Build history of the part. All positions in model axes, mm. A direction names the side the tool comes from. Coordinates: 2 decimals unless noted, no trailing zeros. Loops run counter-clockwise (first coordinate to the right, second up) from the corner with the lowest first, then second, coordinate; pieces in that order, holes last.
Item 1: Mould opens along X. For faces 4 (the face through (114.99, 21, -26)), 5 (the face through (47, 21, -72)), 6 (the face through (92.5, 6, -33)) say: released by +X, released by -X, zero draft, split by the parting line, or undercut.
Item 2: Drill centre lines: line 1 along X through (y, z) = (16.75, -8); line 2 along Z through (x, y) = (46.5, 35); line 3 along Z through (x, y) = (19.5, 8.5). Where is each one in solid material? Low to high.
Item 3: Cut at D-D (y = 25.5). List the corners of the cut face in (x, z).
Item 4: Cut at B-B (z = -14). List the corners of the cut face in (x, y), and give its area (3 significant figures).
Item 5: Cut at A-A (y = 8). List the corners of the cut face in (x, z), and give its area (3 significant figures).
Item 6: Cut at C-C (x = 23.5). List the corners of the cut face in (y, z), and give its area (3 significant figures).
Item 7: Flat gauge pins, fed straight in: pin 1 (1 mm diameter, centred on x = 28, z = -8, fed in from +Y); pin 2 (4 mm diameter, centred on x = 46.5, z = 3.5, fed in from -Y); pin 3 (2.5 mm diameter, centred on x = 0, z = -6, fed in from -Y). Where does each tip first touch, or does it go through?
Item 8: 3-axis set-ups, long thin cutter, end or side, ignore diameter. For faces 1 (the face through (-9.581, 3.042, -0.864)), 2 (the face through (88.026, 16.768, -57.481)), 3 (the face through (111.441, 33.234, -35.2)): which of +Z, -Z, +X, -X, +Y, -Y reach the whole face in a straight line?
Autodesk Inventor part; units mm, degrees
ref_plane "Work Plane2" through (0, 18, 0) normal (0, 1, 0) x (1, 0, 0)
ref_plane "YZ Plane" through (0, 0, 0) normal (1, 0, 0) x (0, 1, 0)
ref_plane "XZ Plane" through (0, 0, 0) normal (0, 1, 0) x (-1, 0, 0)
sketch "Sketch1" plane through (0, 0, 0) normal (0, 1, 0) x (-1, 0, 0)
  line L0 (0, 0) -> (-95, 0)
  line L1 (-95, 0) -> (-95, -65)
  line L2 (-95, -65) -> (0, -65)
  line L3 (0, -65) -> (0, 0)
  line L4 (0, -65) -> (12.9904, -57.5)
  line L5 (12.9904, -57.5) -> (12.9904, -7.5)
  line L6 (12.9904, -7.5) -> (0, 0)
  line L7 (-95, -65) -> (-107.9904, -57.5)
  line L8 (-107.9904, -57.5) -> (-107.9904, -7.5)
  line L9 (-107.9904, -7.5) -> (-95, 0)
  dimension "d0" = 95
  dimension "d1" = 65
  dimension "d2" = 15
  dimension "d3" = 15
  dimension "d4" = 120
  dimension "d5" = 15
  dimension "d6" = 15
  dimension "d7" = 120
extrude "Extrusion1" add sketch "Sketch1" along normal blind 5
sketch "Sketch2" plane through (0, 5, 0) normal (0, 1, 0) x (1, 0, 0)
  line L0 (1.0001, 63.5) -> (94.0001, 63.5)
  line L1 (94.0001, 63.5) -> (94.0001, 1.5)
  line L2 (94.0001, 1.5) -> (1.0001, 1.5)
  line L3 (1.0001, 1.5) -> (1.0001, 63.5)
  line L4 (0, 0) -> (95, 0)
  line L5 (-12.9904, 57.5) -> (-12.9904, 7.5)
  dimension "d10" = 93
  dimension "d11" = 62
  dimension "d12" = 1.5
  dimension "d13" = 13.9905
extrude "Extrusion2" add sketch "Sketch2" along normal blind 8
sketch "Sketch4" plane through (0, 5, 0) normal (0, 1, 0) x (1, 0, 0)
  line L0 (-12.9904, 57.5) -> (-12.9904, 7.5)
  line L1 (-12.9904, 57.5) -> (-12.9904, 7.5)
  line L2 (-12.9904, 7.5) -> (0, 0)
  line L3 (0, 0) -> (95, 0)
  line L4 (95, 0) -> (107.9904, 7.5)
  line L5 (95, 0) -> (107.9904, 7.5)
  line L6 (107.9904, 7.5) -> (107.9904, 57.5)
  line L7 (107.9904, 57.5) -> (95, 65)
  line L8 (107.9904, 57.5) -> (95, 65)
  line L9 (95, 65) -> (0, 65)
  line L10 (95, 65) -> (0, 65)
  line L11 (0, 65) -> (-12.9904, 57.5)
  line L12 (-19.9904, 61.5415) -> (-19.9904, 3.4585)
  line L13 (114.9904, 61.5415) -> (114.9904, 3.4585)
  line L14 (-1.8756, 72) -> (96.8756, 72)
  line L15 (-19.9904, 61.5415) -> (-1.8756, 72)
  line L16 (96.8756, 72) -> (114.9904, 61.5415)
  line L17 (114.9904, 3.4585) -> (96.8756, -7)
  line L18 (-19.9904, 3.4585) -> (-1.8756, -7)
  line L19 (-1.8756, -7) -> (96.8756, -7)
  line L20 (95, 0) -> (107.9904, 7.5)
  line L21 (107.9904, 7.5) -> (107.9904, 57.5)
  line L22 (0, 0) -> (95, 0)
  dimension "d22" = 7
  dimension "d23" = 7
  dimension "d24" = 7
  dimension "d25" = 7
  dimension "d26" = 7
  dimension "d27" = 7
  dimension "d28" = 7
  dimension "d29" = 7
extrude "Extrusion4" add sketch "Sketch4" along normal blind 32 and the other way blind 5
sketch "Sketch5" plane through (0, 0, 0) normal (0, -1, 0) x (1, 0, 0)
  line L0 (2.4999, -63) -> (92.4999, -63)
  line L1 (92.4999, -63) -> (92.4999, -2)
  line L2 (92.4999, -2) -> (2.4999, -2)
  line L3 (2.4999, -2) -> (2.4999, -63)
  line L4 (0, 0) -> (95, 0)
  line L5 (-12.9904, -57.5) -> (-12.9904, -7.5)
  line L6 (96.8756, 7) -> (-1.8756, 7)
  line L7 (114.9904, -61.5415) -> (114.9904, -3.4585)
  line L8 (-1.8756, -72) -> (96.8756, -72)
  dimension "d34" = 61
  dimension "d35" = 90
  dimension "d44" = 22.4905
  dimension "d128" = 9
extrude "Extrusion5" cut sketch "Sketch5" against normal blind 11
chamfer "Chamfer1" distance 6 angle 45 8 edges at (47.5, 0, -72) (105.933, 0, -66.7707) (114.9904, 0, -32.5) (105.933, 0, 1.7707) (47.5, 0, 7) (-10.933, 0, 1.7707) (-19.9904, 0, -32.5) (-10.933, 0, -66.7707)
sketch "Sketch6" plane through (0, 0, 0) normal (0, -1, 0) x (1, 0, 0)
  line L0 (2.4999, -2) -> (-2.5001, -2)
  line L1 (-2.5001, -2) -> (-2.5001, -63.0139)
  line L2 (-2.5001, -63.0139) -> (2.4999, -63.0139)
  line L3 (2.4999, -63.0139) -> (2.4999, -2)
  line L4 (2.4999, -2) -> (92.4999, -2)
  line L5 (92.4999, -2) -> (97.4999, -2)
  line L6 (97.4999, -2) -> (97.4999, -63.0139)
  line L7 (97.4999, -63.0139) -> (92.4999, -63.0139)
  line L8 (92.4999, -63.0139) -> (92.4999, -2)
  point P0 (0, 0)
  dimension "d45" = 5
  dimension "d46" = 5
extrude "Extrusion6" cut sketch "Sketch6" against normal blind 2
sketch "Sketch7" plane through (0, 2, 0) normal (0, -1, 0) x (1, 0, 0)
  circle A0 centre (-0.0001, -6) radius 1.6
  circle A1 centre (94.9999, -6) radius 1.6
  circle A2 centre (-0.0001, -59.0139) radius 1.6
  circle A3 centre (94.9999, -59.0139) radius 1.6
  line L0 (94.0001, -63.5) -> (94.0001, -1.5)
  line L1 (2.4999, -2) -> (2.4999, -63)
  line L2 (97.4999, -2) -> (97.4999, -63.0139)
  line L3 (-2.5001, -2) -> (97.4999, -2)
  line L4 (-2.5001, -63.0139) -> (-2.5001, -2)
  line L5 (2.4999, -63.0139) -> (-2.5001, -63.0139)
  line L6 (92.4999, -63) -> (92.4999, -2)
  line L7 (97.4999, -63.0139) -> (92.4999, -63.0139)
  point P0 (0, 0)
  dimension "d49" = 3.2
  dimension "d50" = 2.5
  dimension "d51" = 2.5
  dimension "d52" = 4
  dimension "d53" = 0
  dimension "d54" = 2.5
  dimension "d55" = 4
  dimension "d56" = 2.5
  dimension "d57" = 4
extrude "Extrusion7" cut sketch "Sketch7" against normal blind 1 contours A0 | A1 L0 | L0 A1 | L0 A3 | A3 L0 | A2
sketch "Sketch8" plane through (0, 13, 0) normal (0, 1, 0) x (1, 0, 0)
  line L0 (5.0001, 60.5) -> (90.0001, 60.5)
  line L1 (90.0001, 60.5) -> (90.0001, 4.5)
  line L2 (90.0001, 4.5) -> (5.0001, 4.5)
  line L3 (5.0001, 4.5) -> (5.0001, 60.5)
  line L4 (96.8756, 72) -> (-1.8756, 72)
  line L5 (-19.9904, 61.5415) -> (-19.9904, 3.4585)
  circle A0 centre (28.5001, 57) radius 2.5
  circle A1 centre (28.5001, 8) radius 2.5
  circle A2 centre (86.5001, 57) radius 2.5
  circle A3 centre (86.5001, 8) radius 2.5
  circle A4 centre (28.5001, 8) radius 1.6
  circle A5 centre (86.5001, 8) radius 1.6
  circle A6 centre (86.5001, 57) radius 1.6
  circle A7 centre (28.5001, 57) radius 1.6
  circle A8 centre (28.5001, 57) radius 2.5
  point P0 (0, 0)
  dimension "d60" = 85
  dimension "d61" = 56
  dimension "d62" = 11.5
  dimension "d63" = 24.9905
  dimension "d65" = 3.5
  dimension "d66" = 5
  dimension "d68" = 3.5
  dimension "d69" = 3.5
  dimension "d70" = 3.5
  dimension "d71" = 58
  dimension "d72" = 58
  dimension "d75" = 3.5
  dimension "d76" = 3.5
  dimension "d100" = 3.2
  dimension "d101" = 3.2
  dimension "d102" = 3.2
  dimension "d103" = 3.2
extrude "Extrusion8" add sketch "Sketch8" along normal blind 5 contours A0 | A1 | A2 | A3 | A4 | A5 | A6 | A7
sketch "Sketch9" plane through (92.4999, 11, -63) normal (-1, 0, 0) x (0, 0, 1)
  circle A0 centre (49, -3) radius 1.5
  line L0 (61, 0) -> (0, 0)
  line L1 (61, -9) -> (61, 0)
  point P0 (63, -11)
  dimension "d77" = 3
  dimension "d78" = 3
  dimension "d79" = 12
extrude "Extrusion9" cut sketch "Sketch9" against normal blind 5
sketch "Sketch10" plane through (0, 37, 0) normal (0, 1, 0) x (1, 0, 0)
  line L0 (-12.9904, 7.5) -> (-12.9904, 57.5)
  line L1 (-12.9904, 7.5) -> (-16.4904, 1.4378)
  line L2 (-1.8756, -7) -> (-19.9904, 3.4585)
  line L3 (0, 0) -> (95, 0)
  line L4 (0, 0) -> (-3.486, -6.038)
  line L5 (-12.9904, 57.5) -> (0, 65)
  line L6 (-12.9904, 57.5) -> (-16.4904, 63.5622)
  line L7 (-1.8756, 72) -> (-19.9904, 61.5415)
  line L8 (0, 65) -> (-3.5, 71.0622)
  line L9 (0, 65) -> (95, 65)
  line L10 (95, 65) -> (98.5, 71.0622)
  line L11 (114.9904, 61.5415) -> (96.8756, 72)
  line L12 (107.9904, 57.5) -> (95, 65)
  line L13 (107.9904, 57.5) -> (111.4904, 63.5622)
  line L14 (95, 0) -> (107.9904, 7.5)
  line L15 (107.9904, 7.5) -> (111.4904, 1.4378)
  line L16 (95, 0) -> (98.5, -6.0622)
  line L17 (96.8756, -7) -> (114.9904, 3.4585)
  circle A0 centre (103.2452, 0.7189) radius 1.6
  circle A1 centre (103.2452, 64.2811) radius 1.6
  circle A2 centre (-8.2452, 64.2811) radius 1.6
  circle A3 centre (-8.2452, 0.7189) radius 1.6
  circle A4 centre (46.5, -3.5) radius 1.6
  circle A5 centre (46.5, 68.5) radius 1.6
  line L18 (0, 0) -> (-12.9904, 7.5)
  line L19 (-12.9904, 7.5) -> (0, 0)
  line L20 (0, 0) -> (0, -7)
  line L21 (-1.8756, -7) -> (96.8756, -7)
  line L22 (0, 65) -> (0, 72)
  dimension "d82" = 3.2
  dimension "d83" = 7.5
  dimension "d84" = 90
  dimension "d85" = 3.5
  dimension "d86" = 90
  dimension "d87" = 7.5
  dimension "d88" = 3.5
  dimension "d89" = 7.5
  dimension "d90" = 3.5
  dimension "d91" = 7.5
  dimension "d92" = 3.5
  dimension "d93" = 46.5
  dimension "d95" = 46.5
  dimension "d96" = 3.5
  dimension "d97" = 3.5
extrude "Extrusion10" cut sketch "Sketch10" against normal blind 3 contours A0 | A1 | A2 | A3 | A4 | A5
ref_plane "Work Plane2" through (0, 18, 0) normal (0, 1, 0) x (1, 0, 0)
sketch "Sketch14" plane through (0, 18, 0) normal (0, 1, 0) x (1, 0, 0)
  circle A0 centre (28.5001, 8) radius 1.6
  circle A1 centre (28.5001, 8) radius 2.5
  line L0 (28.5001, 8) -> (86.5001, 8)
  line L1 (86.5001, 8) -> (86.5001, 64)
  line L2 (86.5001, 64) -> (28.5001, 64)
  line L3 (28.5001, 64) -> (28.5001, 8)
  point P0 (0, 0)
  dimension "d108" = 3.2
  dimension "d109" = 0
  dimension "d110" = 0
  dimension "d117" = 56
  dimension "d118" = 58
extrude "Extrusion11" cut sketch "Sketch14" against normal blind 2.5 contours L0 L3 A0 | A0 L3 L0
sketch "Sketch15" plane through (86.5001, 18, -8) normal (0, 1, 0) x (1, 0, 0)
  circle A0 centre (0, 0) radius 1.6
  circle A1 centre (0, 49) radius 1.6
  circle A2 centre (0, 49) radius 2.5
  circle A3 centre (-58, 0) radius 1.6
  line L0 (-58, 0) -> (0, 0)
  line L1 (0, 0) -> (0, 49)
  line L2 (0, 49) -> (-58, 49)
  line L3 (-58, 49) -> (-58, 0)
  circle A4 centre (-58, 49) radius 1.6
  point P0 (-86.5001, -8)
  dimension "d113" = 3.2
  dimension "d114" = 3.2
  dimension "d115" = 5
  dimension "d116" = 0
  dimension "d119" = 49
  dimension "d120" = 58
  dimension "d121" = 3.2
extrude "Extrusion12" cut sketch "Sketch15" against normal blind 2.5 contours A0 L0 L1 | L1 L0 A0 | L1 L2 A1 | A1 L2 L1 | A4 L3 L2 | L2 L3 A4
sketch "Sketch16" plane through (107.9904, 5, -57.5) normal (-1, 0, 0) x (0, 0, 1)
  circle A0 centre (23.3152, 20.5) radius 7.8
  line L0 (0, 32) -> (50, 32)
  line L1 (0, 32) -> (50, 32)
  line L2 (57.5, 0) -> (50, 0)
  line L3 (50, 32) -> (50, 0)
  line L4 (50, 0) -> (0, 0)
  line L5 (0, 0) -> (0, 32)
  line L6 (0, 0) -> (0, 32)
  line L7 (-52.9421, -1.2141) -> (6.8536, -5)
  line L8 (6.8536, -5) -> (-57.6878, -5)
  line L9 (-57.6878, -5) -> (10.0174, -1.2141)
  point P0 (57.5, -5)
  dimension "d124" = 15.6
  dimension "d125" = 11.5
extrude "Extrusion13" cut sketch "Sketch16" against normal blind 10 contours A0
properties part number "Bottomv5"
Filled sheet:
1. face 4: released by +X
1. face 5: zero draft
1. face 6: undercut
2. line 1: x = -19.99 to -12.99, 26 to 26.9, 30.1 to 31, 84 to 84.9, 88.1 to 89, 107.99 to 114.99
2. line 2: z = -72 to -70.1, -66.9 to -65, 0 to 1.9, 5.1 to 7
2. line 3: z = -72 to -65, -63.5 to -63, -2 to -1.5, 0 to 7
3. outline: (-19.99, -61.54) - (-1.88, -72) - (96.88, -72) - (114.99, -61.54) - (114.99, -41.98) - (107.99, -41.98) - (107.99, -57.5) - (95, -65) - (0, -65) - (-12.99, -57.5) - (-12.99, -7.5) - (0, 0) - (95, 0) - (107.99, -7.5) - (107.99, -26.38) - (114.99, -26.38) - (114.99, -3.46) - (96.88, 7) - (-1.88, 7) - (-19.99, -3.46) - close
4. outline: (-19.99, 6) - (-13.99, 0) - (-2.5, 0) - (-2.5, 2) - (2.5, 2) - (2.5, 11) - (92.5, 11) - (92.5, 9.5) - (94, 9.5) - (94, 13) - (1, 13) - (1, 5) - (-12.99, 5) - (-12.99, 37) - (-19.99, 37) - close; (92.5, 2) - (97.5, 2) - (97.5, 0) - (108.99, 0) - (114.99, 6) - (114.99, 37) - (107.99, 37) - (107.99, 5) - (94, 5) - (94, 6.5) - (92.5, 6.5) - close
4. area: 816 mm2
5. outline: (-19.99, -61.54) - (-1.88, -72) - (96.88, -72) - (114.99, -61.54) - (114.99, -3.46) - (96.88, 7) - (-1.88, 7) - (-19.99, -3.46) - close; (1, -63.5) - (94, -63.5) - (94, -15.5) - (92.5, -15.5) - (92.5, -63) - (2.5, -63) - (2.5, -2) - (92.5, -2) - (92.5, -12.5) - (94, -12.5) - (94, -1.5) - (1, -1.5) - close; hole (-12.99, -57.5) - (0, -65) - (95, -65) - (107.99, -57.5) - (107.99, -7.5) - (95, 0) - (0, 0) - (-12.99, -7.5) - close
5. area: 2,890 mm2
6. outline: (0, -66) - (6, -72) - (37, -72) - (37, -65) - (5, -65) - (5, -63.5) - (13, -63.5) - (13, -1.5) - (5, -1.5) - (5, 0) - (37, 0) - (37, 7) - (6, 7) - (0, 1) - (0, -2) - (11, -2) - (11, -63) - (0, -63) - close
6. area: 632 mm2
7. pin 1: stops at y = 15.5
7. pin 2: stops at y = 0.5
7. pin 3: stops at y = 3
8. face 1: +Z, -X, -Y
8. face 2: +Y
8. face 3: +X
